from build123d import *

# Parameters (mm, degrees)
BOSS_EXTRUDE1_DEPTH = 2.9
SKETCH2_R           = 3.5
CUT_EXTRUDE1_DEPTH  = 3.9


with BuildPart() as part:
    # Sketch1 → Boss-Extrude1 (new body)
    with BuildSketch(Plane(origin=(0, 0, 0), x_dir=(0, 0, -1), z_dir=(1, 0, 0))):
        with BuildLine():
            Line((247.65, -203.2), (277.65, -203.2))
            Line((277.65, -203.2), (277.65, -118.2))
            Line((277.65, -118.2), (280.55, -118.2))
            Line((280.55, -118.2), (280.55, -93.2))
            Line((280.55, -93.2), (277.65, -93.2))
            Line((277.65, -93.2), (277.65, 118.2))
            Line((277.65, 118.2), (280.55, 118.2))
            Line((280.55, 118.2), (280.55, 143.2))
            Line((280.55, 143.2), (277.65, 143.2))
            Line((277.65, 143.2), (277.65, 203.2))
            Line((277.65, 203.2), (-277.65, 203.2))
            Line((-277.65, 203.2), (-277.65, 143.2))
            Line((-277.65, 143.2), (-280.55, 143.2))
            Line((-280.55, 143.2), (-280.55, 118.2))
            Line((-280.55, 118.2), (-277.65, 118.2))
            Line((-277.65, 118.2), (-277.65, -93.2))
            Line((-277.65, -93.2), (-280.55, -93.2))
            Line((-280.55, -93.2), (-280.55, -118.2))
            Line((-280.55, -118.2), (-277.65, -118.2))
            Line((-277.65, -118.2), (-277.65, -203.2))
            Line((-277.65, -203.2), (-247.65, -203.2))
            ThreePointArc((-247.65, -203.2), (-240.578932188, -200.271067812), (-237.65, -193.2))
            Line((-237.65, -193.2), (-237.65, -188.2))
            ThreePointArc((-237.65, -188.2), (-234.721067812, -181.128932188), (-227.65, -178.2))
            Line((-227.65, -178.2), (227.65, -178.2))
            ThreePointArc((227.65, -178.2), (234.721067812, -181.128932188), (237.65, -188.2))
            Line((237.65, -188.2), (237.65, -193.2))
            ThreePointArc((237.65, -193.2), (240.578932188, -200.271067812), (247.65, -203.2))
        make_face()
    extrude(amount=BOSS_EXTRUDE1_DEPTH)

    # Sketch2 → Cut-Extrude1 (cut, through all)
    with BuildSketch(Plane(origin=(2.9, 0, 0), x_dir=(0, 0, -1), z_dir=(1, 0, 0))):
        with Locations((-257.65, 193.2)):
            Circle(SKETCH2_R)
        with Locations((257.65, 193.2)):
            Circle(SKETCH2_R)
    extrude(amount=-CUT_EXTRUDE1_DEPTH, mode=Mode.SUBTRACT)


solid = part.part
Design review of the part built by this model. Coordinates are the model's own, in mm. Coordinates: 2 decimals unless noted, no trailing zeros. Write each loop counter-clockwise with the first axis right and the second up, starting at its lowest first coordinate (ties: lowest second). Pieces come first, ordered by that corner, then holes. Notation, with made-up numbers: (33.5, 1.5) - (76.5, 1.5) arc R22 cw to (76.5, 20.5) - close; hole circle Ø9 at (-2, 41). An arc over 180 degrees is marked (long way). Use one line per item in the form item = value.
Q1. Consider section B-B (z = -32). Write out the cut boundary in (x, y).
Taken from the geometry:
outline = (0, -178.2) - (2.9, -178.2) - (2.9, 203.2) - (0, 203.2) - close
Q2. Insertion check: pin 1 Ø1.5 at (x, z) = (2.5, 136) entering from -Y; pin 2 Ø0.9 at (x, y) = (2, -190) entering from +Z; pin 3 Ø1.4 at (x, z) = (1.5, 279) entering from +Y; pin 4 Ø3 at (y, z) = (-123, 91) entering from -X. Each pin has a flat end and moves straight along its axis. Give the tip position at first contact, or say it passes through.
Taken from the geometry:
pin_1 = -178.2
pin_2 = 277.65
pin_3 = 143.2
pin_4 = 0
Q3. Consider section A-A (x = 1.4). Count the separate pieces of the cut face and the enclosed holes in it, plus the area to 3 significant figures.
Taken from the geometry:
separate_pieces = 1
enclosed_holes = 2
area = 214,000 mm^2
Q4. For probe 1 along Z at (x, y) = (0.9, 193.2); probe 2 along Y at (x, z) = (0.7, -257.65); probe 3 along Y at (x, z) = (2.5, -137), list the stretches that pass through material, from the lowest coordinate up.
Taken from the geometry:
probe_1 = -277.65 to -261.15, -254.15 to 254.15, 261.15 to 277.65
probe_2 = -203.2 to 189.7, 196.7 to 203.2
probe_3 = -178.2 to 203.2
